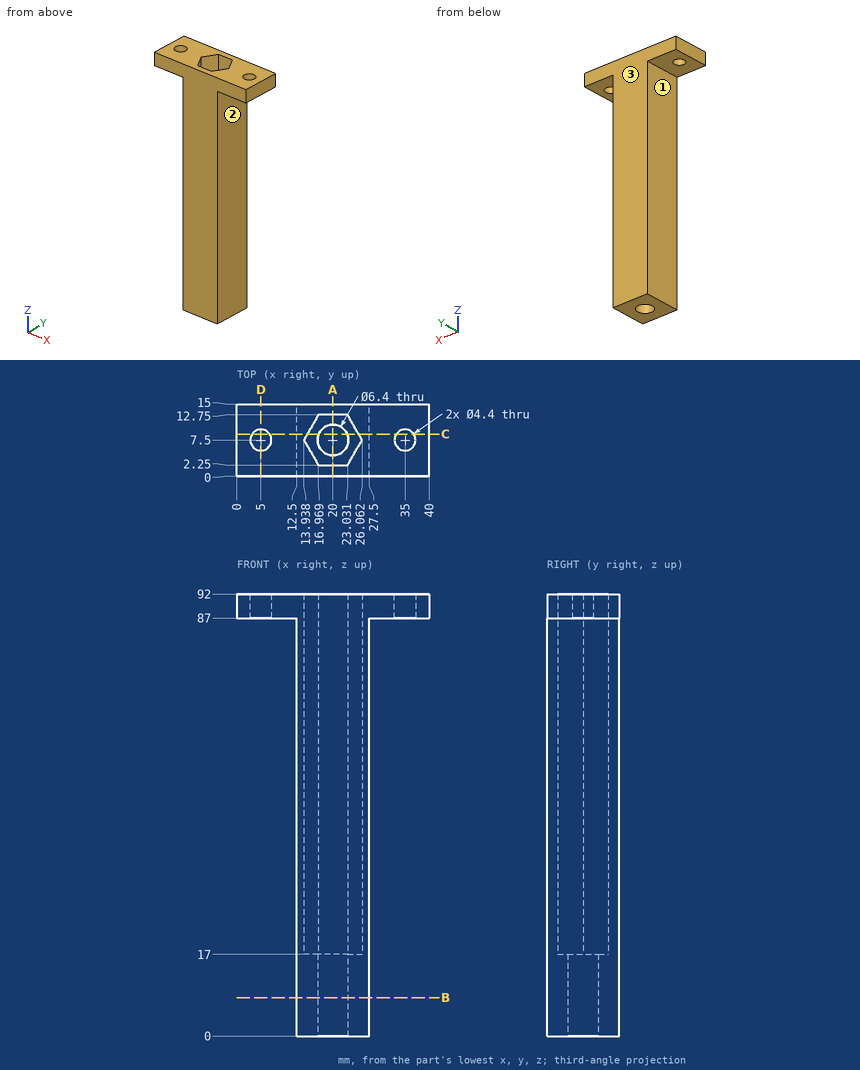
Could you check a few things on this drawing? It's one solid part, dimensions in mm from its lowest x, y, z. A direction names the side the tool comes from. Round coordinates to 2 decimals unless told otherwise and drop trailing zeros. Order: outer loops, then holes, each group sorted by start corner. A loop starts at its lowest first (then second) coordinate and runs counter-clockwise, first axis right, second up.
Q1. Imagine slicing it at A-A, the plane x = 20. List the corners of the cut face in (y, z) for me, then the cut area to 3 significant figures.
Geometry says:
outline: (0, 0) - (4.3, 0) - (4.3, 17) - (2.25, 17) - (2.25, 92) - (0, 92) - close; (10.7, 0) - (15, 0) - (15, 92) - (12.75, 92) - (12.75, 17) - (10.7, 17) - close
area: 484 mm2
Q2. Please list where these lines run through material, in increasing order: probe 1 along Y at (x, z) = (5, 88.1); probe 2 along Y at (x, z) = (18, 71); probe 3 along Z at (x, y) = (36, 13).
Geometry says:
probe 1: y = 0 to 5.3, 9.7 to 15
probe 2: y = 0 to 2.25, 12.75 to 15
probe 3: z = 87 to 92
Q3. Imagine slicing it at B-B, the plane z = 8. List the corners of the cut face in (x, y) for me.
Geometry says:
outline: (12.5, 0) - (27.5, 0) - (27.5, 15) - (12.5, 15) - close; hole circle Ø6.4 at (20, 7.5)
Q4. Imagine slicing it at C-C, the plane y = 8.75. List the corners of the cut face in (x, z) for me.
Geometry says:
outline: (0, 87) - (3.19, 87) - (3.19, 92) - (0, 92) - close; (6.81, 87) - (12.5, 87) - (12.5, 0) - (17.05, 0) - (17.05, 17) - (14.66, 17) - (14.66, 92) - (6.81, 92) - close; (22.95, 0) - (27.5, 0) - (27.5, 87) - (33.19, 87) - (33.19, 92) - (25.34, 92) - (25.34, 17) - (22.95, 17) - close; (36.81, 87) - (40, 87) - (40, 92) - (36.81, 92) - close
Q5. Imagine slicing it at D-D, the plane x = 5. List the corners of the cut face in (y, z) for me, then the cut area to 3 significant figures.
Geometry says:
outline: (0, 87) - (5.3, 87) - (5.3, 92) - (0, 92) - close; (9.7, 87) - (15, 87) - (15, 92) - (9.7, 92) - close
area: 53.0 mm2
Q6. Which directions (+Z, -Z, +X, -X, +Y, -Y) give clear straight access to the entire face, cutting with the end or side of a thin tool? Please do the marked faces 1, 2 and 3.
Geometry says:
face 1: -Z, -X, +Y, -Y
face 2: -Z, +X, +Y, -Y
face 3: +Z, -Z, +X, -X, +Y
Q7. I'm going to push flat-ended pins straight in: P1, Ø1.5, axis at y = 8.5, z = 20.5, coming from the +X side; P2, Ø5, axis at y = 10, z = 67, coming from the -X side; P3, Ø5, axis at x = 21, y = 8.5, coming from the +Z side; P4, Ø3.5, axis at x = 5, y = 7.5, coming from the -Z side. Where does each tip first touch, or does it pass through?
Geometry says:
P1: stops at x = 27.5
P2: stops at x = 12.5
P3: stops at z = 17
P4: passes through
